For this review, take the finished solid that the model builds, in its own axes (mm). Coordinates: 2 decimals unless noted, no trailing zeros. Order: outer loops, then holes, each group sorted by start corner. A loop starts at its lowest first (then second) coordinate and runs counter-clockwise, first axis right, second up.
from build123d import *

# Parameters (mm, degrees)
SKETCH1_W           = 100
SKETCH1_H           = 100
SKETCH1_R           = 2.5
BOSS_EXTRUDE1_DEPTH = 6
FILLET1_R           = 3
FILLET2_R           = 3
SCALE1_SCALE        = 7.5


with BuildPart() as part:
    # Sketch1 → Boss-Extrude1 (new body)
    with BuildSketch(Plane(origin=(0, 0, 0), x_dir=(1, 0, 0), z_dir=(0, 1, 0))):
        with Locations((40, 40)):
            Rectangle(SKETCH1_W, SKETCH1_H)
        Circle(SKETCH1_R, mode=Mode.SUBTRACT)
        with Locations((80, 0)):
            Circle(SKETCH1_R, mode=Mode.SUBTRACT)
        with Locations((0, 80)):
            Circle(SKETCH1_R, mode=Mode.SUBTRACT)
        with Locations((80, 80)):
            Circle(SKETCH1_R, mode=Mode.SUBTRACT)
        with Locations((22, 22)):
            Circle(SKETCH1_R, mode=Mode.SUBTRACT)
        with Locations((58, 22)):
            Circle(SKETCH1_R, mode=Mode.SUBTRACT)
        with Locations((22, 54)):
            Circle(SKETCH1_R, mode=Mode.SUBTRACT)
        with Locations((58, 54)):
            Circle(SKETCH1_R, mode=Mode.SUBTRACT)
    extrude(amount=BOSS_EXTRUDE1_DEPTH)

    # Fillet1
    fillet1_edges = [part.edges().sort_by_distance(p)[0] for p in [
        (90, 3, 10),
        (-10, 3, 10),
    ]]
    fillet(fillet1_edges, radius=FILLET1_R)

    # Fillet2
    fillet2_edges = [part.edges().sort_by_distance(p)[0] for p in [
        (-10, 3, -90),
        (90, 3, -90),
    ]]
    fillet(fillet2_edges, radius=FILLET2_R)


with BuildPart() as part_1:
    # Scale1: scaled about (40, 3, -40.015971177)
    add(part.part.scale(SCALE1_SCALE).moved(Location((-260, -19.5, 260.103812651))))


solid = part_1.part
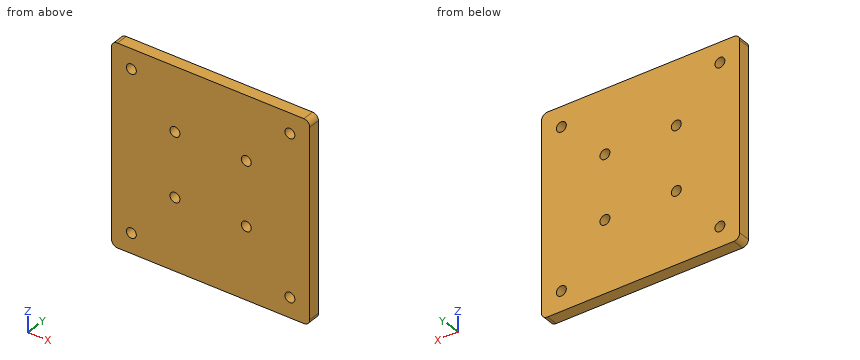
1. Take a section at B-B, the plane y = -7. Give the number of separate pieces and of enclosed holes in the cut face, plus the area to 3 significant figures.
Answer below:
separate pieces: 1
enclosed holes: 8
area: 553,000 mm2
2. Take a section at A-A, the plane x = -260. Give the boundary of the cut face in (y, z).
Answer below:
outline: (-19.5, -414.9) - (25.5, -414.9) - (25.5, -358.65) - (-19.5, -358.65) - close; (-19.5, -321.15) - (25.5, -321.15) - (25.5, 241.35) - (-19.5, 241.35) - close; (-19.5, 278.85) - (25.5, 278.85) - (25.5, 335.1) - (-19.5, 335.1) - close
3. To check wall thickness, follow L1, parallel to Z at x = -260, y = -1; L2, parallel to Z at x = -95, y = -2; L3, parallel to X at y = 0.5, z = -151.5. State the ranges of each line that lie inside material, in increasing order.
Answer below:
L1: z = -414.9 to -358.65, -321.15 to 241.35, 278.85 to 335.1
L2: z = -414.9 to -163.65, -126.15 to 76.35, 113.85 to 335.1
L3: x = -335 to -112.55, -77.45 to 157.45, 192.55 to 415
